```python
from build123d import *

# Parameters (mm, degrees)
SM_BASE_FLANGE_1_DEPTH = 8
SKETCH_6_R             = 2.15
CUT_EXTRUDE_1_DEPTH    = 45.407206622
CHAMFER_1_SIZE         = 2
SKETCH_7_R             = 2.25
CUT_EXTRUDE_2_DEPTH    = 84.258633186
SKETCH_8_R             = 2.25
CUT_EXTRUDE_3_DEPTH    = 84.258633186


# Sheet-metal steps are written as plain solids
with BuildPart() as part:
    # Sketch 1 → 基体-法兰1 (new body)
    with BuildSketch(Plane(origin=(0, 0, 0), x_dir=(1, 0, 0), z_dir=(0, 1, 0))):
        with BuildLine():
            Line((-40, 10), (-40, 2))
            ThreePointArc((-40, 2), (-39.414213562, 0.585786438), (-38, 0))
            Line((-38, 0), (36, 0))
            ThreePointArc((36, 0), (38.828427125, -1.171572875), (40, -4))
            Line((40, -4), (40, -12))
            Line((40, -12), (38, -12))
            Line((38, -12), (38, -4))
            ThreePointArc((38, -4), (37.414213562, -2.585786438), (36, -2))
            Line((36, -2), (-38, -2))
            ThreePointArc((-38, -2), (-40.828427125, -0.828427125), (-42, 2))
            Line((-42, 2), (-42, 10))
            Line((-42, 10), (-40, 10))
        make_face()
    extrude(amount=SM_BASE_FLANGE_1_DEPTH)

    # 草图6 → 切除-拉伸1 (cut, through all)
    with BuildSketch(Plane.XY.offset(2)):
        with Locations((-22.5, 4)):
            Circle(SKETCH_6_R)
        with Locations((22.5, 4)):
            Circle(SKETCH_6_R)
    extrude(amount=-CUT_EXTRUDE_1_DEPTH, mode=Mode.SUBTRACT)

    # 倒角1
    chamfer_1_edges = [part.edges().sort_by_distance(p)[0] for p in [
        (39, 0, 12),
        (-41, 0, -10),
        (39, 8, 12),
        (-41, 8, -10),
    ]]
    chamfer(chamfer_1_edges, length=CHAMFER_1_SIZE)

    # 草图7 → 切除-拉伸2 (cut, through all)
    with BuildSketch(Plane.ZY.offset(42)):
        with Locations((-6, 4)):
            Circle(SKETCH_7_R)
    extrude(amount=-CUT_EXTRUDE_2_DEPTH, mode=Mode.SUBTRACT)

    # 草图8 → 切除-拉伸3 (cut, through all)
    with BuildSketch(Plane(origin=(40, 0, 0), x_dir=(0, 0, -1), z_dir=(1, 0, 0))):
        with Locations((-8, 4)):
            Circle(SKETCH_8_R)
    extrude(amount=-CUT_EXTRUDE_3_DEPTH, mode=Mode.SUBTRACT)


solid = part.part
```
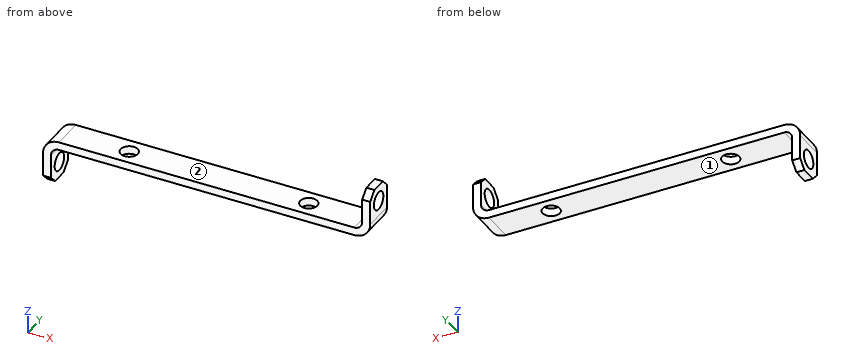
CAD build for the part. Positions are in the model's coordinates, mm. Face numbers are marked on the shaded views. A direction names the side the tool comes from. Round coordinates to 2 decimals unless told otherwise and drop trailing zeros. Order: outer loops, then holes, each group sorted by start corner. A loop starts at its lowest first (then second) coordinate and runs counter-clockwise, first axis right, second up.
Q1. Slice it at D-D (x = 32.5). Write the cut outline in (y, z).
Q2. Which spindle directions (+Z, -Z, +X, -X, +Y, -Y) get a long thin tool onto all of the face, cutting with end or side? Do the marked faces 1 and 2. Say none if no direction does.
Q3. Wall check: L1, parallel to Y at x = -41, z = -6; L2, parallel to Y at x = -22.5, z = 1; L3, parallel to Z at x = -11, y = 3. Give the ranges that are in metal, low to high.
Q4. Slice it at C-C (y = 4). Write the cut outline in (x, z), and give its area (3 significant figures).
Q5. Slice it at A-A (z = -6). Write the cut outline in (x, y).
Q6. Slice it at B-B (x = 22.5). Write the cut outline in (y, z), and give its area (3 significant figures).
Q7. Drop flat-ended pins along their axis: pin 1 (2.5 mm diameter, centred on x = 15, y = 5, fed in from +Z); pin 2 (2.5 mm diameter, centred on x = -22.5, y = 4, fed in from -Z); pin 3 (12 mm diameter, centred on x = 5.5, z = 4.5, fed in from +Y); pin 4 (2 mm diameter, centred on x = 15.5, y = 1, fed in from -Z). Give the stop position or say it passes through.
Results below:
1. outline: (0, 0) - (8, 0) - (8, 2) - (0, 2) - close
2. face 1: -Z, +X, +Y, -Y
2. face 2: +Z, -X, +Y, -Y
3. L1: y = 0 to 1.75, 6.25 to 8
3. L2: y = 0 to 1.85, 6.15 to 8
3. L3: z = 0 to 2
4. outline: (-42, -10) - (-40, -10) - (-40, -8.25) - (-42, -8.25) - close; (-42, -3.75) - (-40, -3.75) - (-40, -2) arc R2 cw to (-38, 0) - (-24.65, 0) - (-24.65, 2) - (-38, 2) arc R4 ccw to (-42, -2) - close; (-20.35, 0) - (20.35, 0) - (20.35, 2) - (-20.35, 2) - close; (24.65, 0) - (36, 0) arc R4 ccw to (40, 4) - (40, 5.75) - (38, 5.75) - (38, 4) arc R2 cw to (36, 2) - (24.65, 2) - close; (38, 10.25) - (40, 10.25) - (40, 12) - (38, 12) - close
4. area: 164 mm2
5. outline: (-42, 0) - (-40, 0) - (-40, 1.75) - (-42, 1.75) - close; (-42, 6.25) - (-40, 6.25) - (-40, 8) - (-42, 8) - close
6. outline: (0, 0) - (1.85, 0) - (1.85, 2) - (0, 2) - close; (6.15, 0) - (8, 0) - (8, 2) - (6.15, 2) - close
6. area: 7.40 mm2
7. pin 1: stops at z = 2
7. pin 2: passes through
7. pin 3: stops at y = 8
7. pin 4: stops at z = 0
